Autodesk Fusion 360 part; units mm, degrees
sketch "Sketch1" plane through (0, 0, 0) normal (0, 1, 0) x (1, 0, 0)
  line L0 (0, 0) -> (0, -40)
  line L1 (0, -40) -> (60, -40)
  line L2 (60, -40) -> (60, 0)
  line L3 (60, 0) -> (0, 0)
  dimension "d1" = 60
  dimension "d2" = 40
  dimension "d3" = 90
  dimension "d4" = 90
extrude "Extrude1" add sketch "Sketch1" along normal blind 1
sketch "Sketch2" plane through (0, 1, 0) normal (0, 1, 0) x (-1, 0, 0)
  line L0 (-60, 0) -> (0, 0)
  line L1 (0, 0) -> (0, 40)
  line L2 (0, 40) -> (-60, 40)
  line L3 (-60, 40) -> (-60, 0)
  line L4 (-24, 8) -> (-39, 8)
  line L5 (-39, 8) -> (-39, 33)
  line L6 (-39, 33) -> (-24, 33)
  line L7 (-24, 33) -> (-24, 8)
  dimension "d18" = 15
  dimension "d19" = 25
  dimension "d20" = 24
  dimension "d21" = 8
extrude "Extrude2" add sketch "Sketch2" along normal blind 10 contours L4 L5 L6 L7
sketch "Sketch3" plane through (0, 11, 0) normal (0, 1, 0) x (-1, 0, 0)
  line L0 (-24, 33) -> (-39, 33)
  line L1 (-39, 33) -> (-39, 8)
  line L2 (-39, 8) -> (-24, 8)
  line L3 (-24, 8) -> (-24, 33)
  line L4 (-25, 9) -> (-38, 9)
  line L5 (-38, 9) -> (-38, 32)
  line L6 (-38, 32) -> (-25, 32)
  line L7 (-25, 32) -> (-25, 9)
  line L8 (-29.5, 8) -> (-29.5, 9)
  line L9 (-33.5, 8) -> (-33.5, 9)
  dimension "d24" = 1
  dimension "d25" = 1
  dimension "d26" = 1
  dimension "d27" = 1
  dimension "d28" = 4
  dimension "d29" = 5.5
extrude "Extrude3" cut sketch "Sketch3" against normal blind 10 contours L2 L4 L8 L9 | L4 L5 L6 L7
sketch "Sketch4" plane through (0, 1, 0) normal (0, 1, 0) x (-1, 0, 0)
  line L0 (-24, 33) -> (-24, 8)
  line L1 (-24, 8) -> (-29.5, 8)
  line L2 (-29.5, 8) -> (-29.5, 9)
  line L3 (-29.5, 9) -> (-25, 9)
  line L4 (-25, 9) -> (-25, 32)
  line L5 (-25, 32) -> (-38, 32)
  line L6 (-38, 32) -> (-38, 9)
  line L7 (-38, 9) -> (-33.5, 9)
  line L8 (-33.5, 9) -> (-33.5, 8)
  line L9 (-33.5, 8) -> (-39, 8)
  line L10 (-39, 8) -> (-39, 33)
  line L11 (-39, 33) -> (-24, 33)
  line L12 (-60, 0) -> (0, 0)
  line L13 (0, 0) -> (0, 40)
  line L14 (0, 40) -> (-60, 40)
  line L15 (-60, 40) -> (-60, 0)
  circle A0 centre (-31.5, 34.5) radius 2
  circle A1 centre (-31.5, 34.5) radius 0.5
  dimension "d32" = 1
  dimension "d33" = 4
  dimension "d35" = 2.5
  dimension "d36" = 6.5
extrude "Extrude4" add sketch "Sketch4" along normal blind 15 contours L11 A0 picked at (-31.4875, 33.3338)
sketch "Sketch5" plane through (0, 0, 0) normal (0, 0, 1) x (1, 0, 0)
extrude "Extrude5" add 1 faces at (31.4875, 16, 33.3338) along direction (0, -1, 0) blind 5
extrude "Extrude6" add 1 faces at (31.059, 11, 32.3333) along direction (0, 1, 0) blind 5
Design review of the part built by this model. Coordinates are the model's own, in mm. A direction names the side the tool comes from. Give positions to 0.01 mm unless a question says otherwise; leave off trailing zeros. Order: outer loops, then holes, each group sorted by start corner. A loop starts at its lowest first (then second) coordinate and runs counter-clockwise, first axis right, second up. Notation, with made-up numbers: (38.25, -24.75) - (57.25, -24.75) arc R16 ccw to (57.25, -17.75) - close; hole circle Ø7 at (56, -17). An arc over 180 degrees is marked (long way). Use a Markdown table: item, result. Add a question column.
(1) Clearance check with flat-ended pins moving along their axes: P1, Ø6, axis at y = 4.5, z = 8.5, coming from the -X side; P2, Ø1.3, axis at x = 36, y = 11.5, coming from the +Z side; P3, Ø4.5, axis at x = 37, y = 11.5, coming from the -Z side. State where each tip first meets the part, or that it passes through.
(2) Machinability: for faces 5 (the face through (36, 8, 9)), 6 (the face through (39, 8, 20)), 7 (the face through (36, 8, 8)), 8 (the face through (30, 0, 20)), which of the approach directions +Z, -Z, +X, -X, +Y, -Y give a long, thin tool a straight path to every point of the face, cutting with its end or side? Answer none if there is none.
(3) Add section B-B on z = 26. Give the boundary of the cut face in (x, y), then the cut area to 3 significant figures.
(4) Wall thickness on probe 1 along X at (y, z) = (4.25, 34.5); probe 2 along X at (y, z) = (2, 14); probe 3 along Z at (x, y) = (31.5, 6.5): over which ranges is each line inside the solid? List them lowest first. Write a range as [from, to].
(5) Add section A-A on y = 15. Give the boundary of the cut face in (x, z).
(6) Mouldability with a two-part tool opening along X and no side actions: class faces 1 (the face through (24, 8, 21)), 2 (the face through (38.2, 16, 22.3)), 3 (the face through (25, 8, 21)), 4 (the face through (30, 1, 20)) as +X half, -X half, draft (parallel to the pull), parting line (faces both ways), or undercut.
(7) Add section C-C on x = 8.5. Give the boundary of the cut face in (y, z).
(8) Add section D-D on z = 5.5. Give the boundary of the cut face in (x, y).
Report:
| question | item | result |
|---|---|---|
| 1 | P1 | stops at x = 24 |
| 1 | P2 | stops at z = 33 |
| 1 | P3 | stops at z = 8 |
| 2 | face 5 | +Y |
| 2 | face 6 | +Z, -Z, +X, +Y |
| 2 | face 7 | -Z, +X, -X, +Y |
| 2 | face 8 | +Z, -Z, +X, -X, -Y |
| 3 | outline | (0, 0) - (60, 0) - (60, 1) - (39, 1) - (39, 16) - (38, 16) - (38, 1) - (25, 1) - (25, 16) - (24, 16) - (24, 1) - (0, 1) - close |
| 3 | area | 90.0 mm² |
| 4 | probe 1 | x = [29.5, 31], [32, 33.5] |
| 4 | probe 2 | x = [24, 25], [38, 39] |
| 4 | probe 3 | z = [32, 34], [35, 36.5] |
| 5 | outline | (24, 8) - (29.5, 8) - (29.5, 9) - (25, 9) - (25, 32) - (38, 32) - (38, 9) - (33.5, 9) - (33.5, 8) - (39, 8) - (39, 33) - (32.82, 33) arc R2 ccw (long way) to (30.18, 33) - (24, 33) - close; hole circle Ø1 at (31.5, 34.5) |
| 6 | face 1 | -X half |
| 6 | face 2 | draft |
| 6 | face 3 | undercut |
| 6 | face 4 | undercut |
| 7 | outline | (0, 0) - (1, 0) - (1, 40) - (0, 40) - close |
| 8 | outline | (0, 0) - (60, 0) - (60, 1) - (0, 1) - close |
